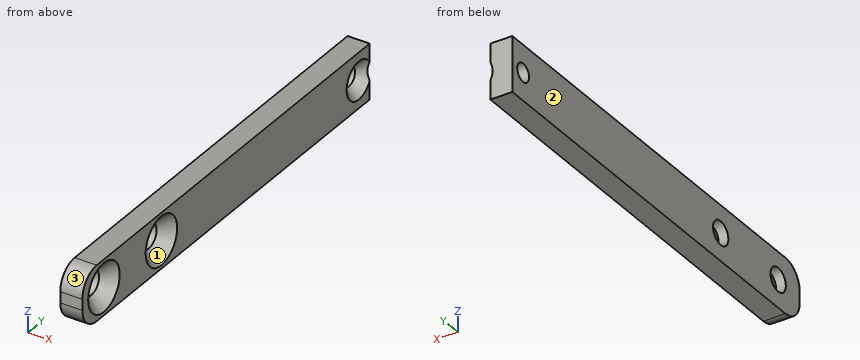
from build123d import *

# Parameters (mm, degrees)
F0_W           = 127
F0_H           = 15.875
F1_DEPTH       = 6.35
F3_D           = 6.7564
F3_CSINK_D     = 13.9192
F3_CSINK_ANGLE = 90
F4_D           = 5.2324
F4_CSINK_D     = 10.8712
F4_CSINK_ANGLE = 90
F5_R           = 6.35


with BuildPart() as f1:
    # F0 (on Right) → F1 (new body)
    with BuildSketch(Plane.YZ):
        with Locations((63.5, 7.9375)):
            Rectangle(F0_W, F0_H)
    extrude(amount=F1_DEPTH)

    # F3 (through all)
    with Locations(Plane.YZ.offset(6.35)):
        with Locations((9.525, 7.9375), (34.925, 7.9375)):
            CounterSinkHole(F3_D / 2, F3_CSINK_D / 2, counter_sink_angle=F3_CSINK_ANGLE)

    # F4 (through all)
    with Locations(Plane.YZ.offset(6.35)):
        with Locations((122.2375, 7.9375)):
            CounterSinkHole(F4_D / 2, F4_CSINK_D / 2, counter_sink_angle=F4_CSINK_ANGLE)

    # F5
    f5_edges = [f1.edges().sort_by_distance(p)[0] for p in [
        (3.175, 0, 15.875),
        (3.175, 0, 0),
    ]]
    fillet(f5_edges, radius=F5_R)


solid = f1.part
Design review of the part built by this model. Coordinates are the model's own, in mm. Face numbers are marked on the shaded views. Coordinates: 2 decimals unless noted, no trailing zeros. Write each question's results on one line, items separated by ' | '. Start each with the question number.
(1) Clearance check with flat-ended pins moving along their axes: P1, Ø9, axis at y = 34.92, z = 7.94, coming from the -X side; P2, Ø2, axis at x = 2, z = 14, coming from the -Y side. State where each tip first meets the part, or that it passes through.
(2) For line 1 along Y through (x, z) = (1.5, 8.25); line 2 along Y through (x, z) = (5.25, 2.75); line 3 along Y through (x, z) = (0.5, 7), list the stretches that pass through material, from the lowest coordinate up. Write a range as from..to.
(3) The part is to be moulded in two halves that separate along Y. For the marked faces 1, 2 and 3, say which applies: pulls with the +Y half, pulls with the -Y half, needs draft (parallel to the pull), parting line crosses it, or undercut.
Results found:
1) P1: stops at x = 0 | P2: stops at y = 1.04
2) line 1: y = 0..6.16, 12.89..31.56, 38.29..119.64, 124.83..127 | line 2: y = 1.12..6.8, 12.25..32.2, 37.65..127 | line 3: y = 0..6.28, 12.77..31.68, 38.17..119.8, 124.68..127
3) face 1: undercut | face 2: needs draft | face 3: pulls with the -Y half
